Could you check a few things on this model? Use its own coordinates, in mm. A direction names the side the tool comes from. Coordinates: 2 decimals unless noted, no trailing zeros. Loops run counter-clockwise (first coordinate to the right, second up) from the corner with the lowest first, then second, coordinate; pieces in that order, holes last.
from build123d import *

# Parameters (mm, degrees)
REVOLVE_1_ANGLE          = 180
HOLE_WIZARD_M3_1_D       = 3.4
HOLE_WIZARD_M3_1_DEPTH   = 5
PATTERN_CIRCULAR_1_COUNT = 4
PATTERN_CIRCULAR_1_ANGLE = 135
MIRROR_1_COPY_1_D        = 3.4
MIRROR_1_COPY_1_DEPTH    = 5
MIRROR_1_COPY_2_D        = 3.4
MIRROR_1_COPY_2_DEPTH    = 5
MIRROR_1_COPY_3_D        = 3.4
MIRROR_1_COPY_3_DEPTH    = 5


with BuildPart() as part:
    # ｽｹｯﾁ1 → 回転1 (revolve)
    with BuildSketch(Plane.XY):
        Polygon((-80, 40), (-50, 40), (-50, 49), (50, 49), (50, 40), (80, 40), (80, 50), (75, 50), (75, 42), (55, 42), (55, 50), (-55, 50), (-55, 42), (-75, 42), (-75, 50), (-80, 50), align=None)
    revolve(axis=Axis((-50, 0, 0), (1, 0, 0)), revolution_arc=REVOLVE_1_ANGLE)

    # M3 すきま穴1
    with Locations(Plane.ZY.offset(80)):
        with Locations((17.220754456, -41.574578963)):
            hole_wizard_m3_1 = Hole(HOLE_WIZARD_M3_1_D / 2, depth=HOLE_WIZARD_M3_1_DEPTH)

    # 円形ﾊﾟﾀｰﾝ1: M3 すきま穴1 ×4 about axis
    pattern_circular_1_axis = Axis((0, 0, 0), (-1, 0, 0))
    for i in range(1, PATTERN_CIRCULAR_1_COUNT):
        add(hole_wizard_m3_1.rotate(pattern_circular_1_axis, i * PATTERN_CIRCULAR_1_ANGLE / (PATTERN_CIRCULAR_1_COUNT - 1)), mode=Mode.SUBTRACT)

    # ﾐﾗｰ1: M3 すきま穴1 across plane
    add(hole_wizard_m3_1.mirror(Plane(origin=(0, 0, 0), x_dir=(0, 0, 1), z_dir=(1, 0, 0))), mode=Mode.SUBTRACT)

    # ﾐﾗｰ1 copy 1
    with Locations(Plane(origin=(80, 0, 0), x_dir=(0, 0.7071067811865487, 0.7071067811865464), z_dir=(1, 0, 0))):
        with Locations((17.220754456, 41.574578963)):
            Hole(MIRROR_1_COPY_1_D / 2, depth=MIRROR_1_COPY_1_DEPTH)

    # ﾐﾗｰ1 copy 2
    with Locations(Plane.YZ.offset(80)):
        with Locations((17.220754456, 41.574578963)):
            Hole(MIRROR_1_COPY_2_D / 2, depth=MIRROR_1_COPY_2_DEPTH)

    # ﾐﾗｰ1 copy 3
    with Locations(Plane(origin=(80, 0, 0), x_dir=(0, 0.7071067811865441, -0.7071067811865509), z_dir=(1, 0, 0))):
        with Locations((17.220754456, 41.574578963)):
            Hole(MIRROR_1_COPY_3_D / 2, depth=MIRROR_1_COPY_3_DEPTH)


solid = part.part
1) If I drill on L1, parallel to X at y = -31, z = 28.5; L2, parallel to X at y = -31.5, z = 26; L3, parallel to Y at x = 1, z = 10, over which ranges is the centre line in solid material (lowest first)?
2) Imagine slicing it at C-C on x = -41. List the corners of the cut face in (y, z) for me.
3) We'd pull the mould along Y, two halves only. Please class faces 1 (the cylindrical face through (-65.14, 0.92, 41.99)), 2 (the cylindrical face through (0.7, 1.08, 48.99)), 3 (the flat face through (-0.4, -49.8, 0)): released by +Y, released by -Y, zero draft, split by the parting line, or undercut.
4) Imagine slicing it at D-D on y = -25.5. List the corners of the cut face in (x, z) for me, plus the area to 3 significant figures.
5) Imagine slicing it at B-B on y = 0. List the corners of the cut face in (x, z) for me, plus the area to 3 significant figures.
6) Will these pins go through, and if not, where does the flat tip stop? pin 1 (2 mm diameter, centred on y = 41.57, z = 17.22, fed in from +X); pin 2 (2 mm diameter, centred on y = 41.57, z = 17.22, fed in from -X); pin 3 (8 mm diameter, centred on x = -9.5, z = 25.5, fed in from -Y).
7) For faces 4 (the cylindrical face through (77.46, 18.57, 40.54)), 5 (the flat face through (-75, -7, 42)), 6 (the flat face through (-50, 4, 41)), 7 (the cylindrical face through (-77.46, -18.01, 40.07)), which set-ups out of +Z, -Z, +X, -X, +Y, -Y let a thin tool reach every point of the face, with its end or its side?
Solved:
1. L1: x = -80 to -75, -55 to -50, 50 to 55, 75 to 80
1. L2: x = -80 to -50, 50 to 80
1. L3: y = -48.99 to -47.97, 47.97 to 48.99
2. outline: (-50, 0) - (-49, 0) arc R49 cw to (49, 0) - (50, 0) arc R50 ccw to start
3. face 1: split by the parting line
3. face 2: undercut
3. face 3: zero draft
4. outline: (-80, 30.82) - (-50, 30.82) - (-50, 41.84) - (50, 41.84) - (50, 30.82) - (80, 30.82) - (80, 43.01) - (75, 43.01) - (75, 33.37) - (55, 33.37) - (55, 43.01) - (-55, 43.01) - (-55, 33.37) - (-75, 33.37) - (-75, 43.01) - (-80, 43.01) - close
4. area: 463 mm2
5. outline: (-80, 40) - (-50, 40) - (-50, 49) - (50, 49) - (50, 40) - (80, 40) - (80, 50) - (75, 50) - (75, 42) - (55, 42) - (55, 50) - (-55, 50) - (-55, 42) - (-75, 42) - (-75, 50) - (-80, 50) - close
5. area: 380 mm2
6. pin 1: stops at x = 55
6. pin 2: stops at x = -55
6. pin 3: stops at y = -45.14
7. face 4: +X
7. face 5: +Z
7. face 6: -Z
7. face 7: -X
